Geometry: see drawing. Coordinates: mm, zero at the bounding-box minimum. Coordinates: 2 decimals unless noted, no trailing zeros. Order: outer loops, then holes, each group sorted by start corner. A loop starts at its lowest first (then second) coordinate and runs counter-clockwise, first axis right, second up.
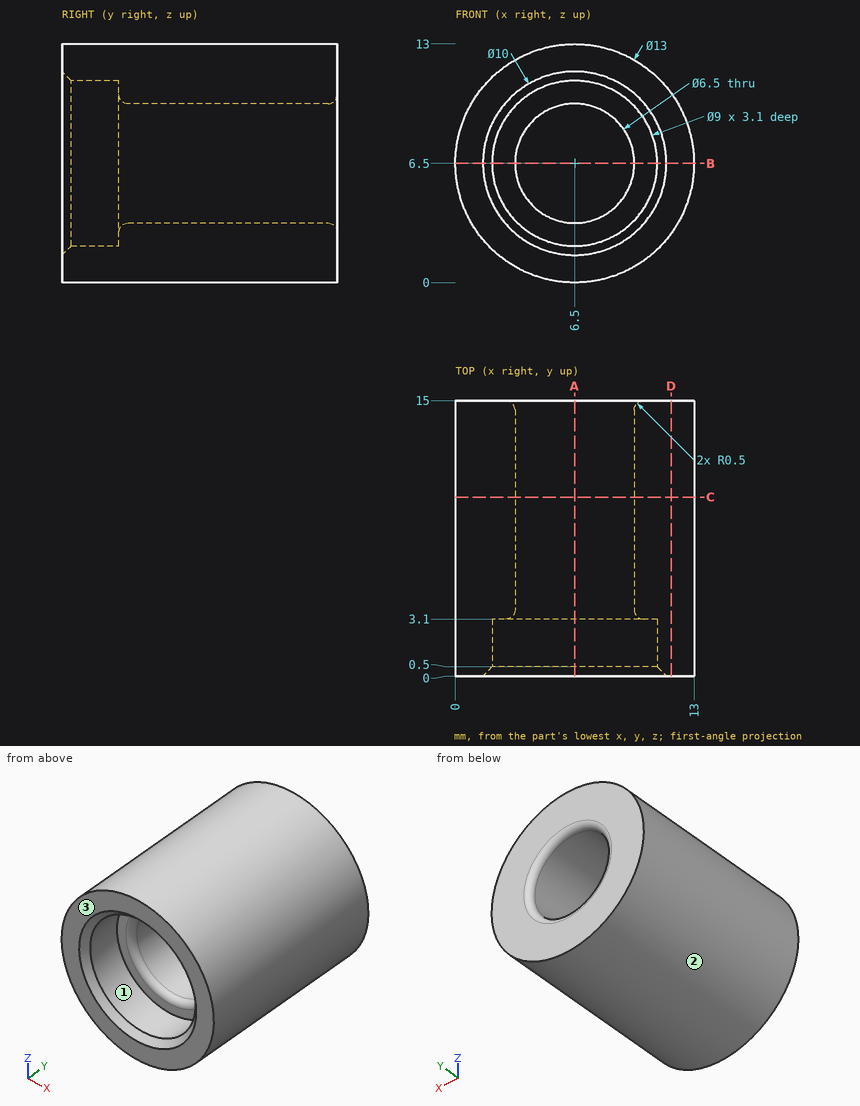
Q1. Material intervals for line 1 along X through (y, z) = (2, 6.5); line 2 along X through (y, z) = (11.5, 6.5); line 3 along Y through (x, z) = (7.75, 10.75), sorted ascending.
Solutions:
line 1: x = 0 to 2, 11 to 13
line 2: x = 0 to 3.25, 9.75 to 13
line 3: y = 3.1 to 15
Q2. Section query A-A on x = 6.5. Output: boundary loops of the cut face in (y, z).
Solutions:
outline: (0, 0) - (15, 0) - (15, 2.75) arc R0.5 ccw to (14.5, 3.25) - (3.6, 3.25) arc R0.5 ccw to (3.1, 2.75) - (3.1, 2) - (0.5, 2) - (0, 1.5) - close; (0, 11.5) - (0.5, 11) - (3.1, 11) - (3.1, 10.25) arc R0.5 ccw to (3.6, 9.75) - (14.5, 9.75) arc R0.5 ccw to (15, 10.25) - (15, 13) - (0, 13) - close
Q3. Section query B-B on z = 6.5. Output: boundary loops of the cut face in (x, y), plus the area to 3 significant figures.
Solutions:
outline: (0, 0) - (1.5, 0) - (2, 0.5) - (2, 3.1) - (2.75, 3.1) arc R0.5 ccw to (3.25, 3.6) - (3.25, 14.5) arc R0.5 ccw to (2.75, 15) - (0, 15) - close; (9.75, 3.6) arc R0.5 ccw to (10.25, 3.1) - (11, 3.1) - (11, 0.5) - (11.5, 0) - (13, 0) - (13, 15) - (10.25, 15) arc R0.5 ccw to (9.75, 14.5) - close
area: 89.3 mm2
Q4. Pin query (flat end, axial travel): P1, Ø7, axis at x = 6.5, z = 6.5, coming from the +Y side; P2, Ø5, axis at x = 9.5, y = 7, coming from the +Z side. Return the tip coordinate at first contact, or that it passes through.
Solutions:
P1: stops at y = 14.93
P2: stops at z = 12.98
Q5. Section query D-D on x = 11.75. Output: boundary loops of the cut face in (y, z), plus the area to 3 significant figures.
Solutions:
outline: (0, 2.67) - (15, 2.67) - (15, 10.33) - (0, 10.33) - close
area: 115 mm2
Q6. Pull-direction query (X, two-part tool) for the marked faces 1, 2 and 3; classes: pulls with the +X half, pulls with the -X half, needs draft (parallel to the pull), parting line crosses it, or undercut.
Solutions:
face 1: undercut
face 2: parting line crosses it
face 3: needs draft
Q7. Section query C-C on y = 9.75. Output: boundary loops of the cut face in (x, z), plus the area to 3 significant figures.
Solutions:
outline: circle Ø13 at (6.5, 6.5); hole circle Ø6.5 at (6.5, 6.5)
area: 99.5 mm2
